Input: part model. Units: mm. Frame: model coordinates. Face numbers are marked on the shaded views. A direction names the side the tool comes from. Coordinates: 2 decimals unless noted, no trailing zeros. Order: outer loops, then holes, each group sorted by start corner. A loop starts at its lowest first (then second) coordinate and runs counter-clockwise, first axis right, second up. Notation, with made-up numbers: M 0,39.25 L 54,39.25 A11 cw 54,57.25 Z; hole C 82,60 d8. An arc over 180 degrees is marked long. Answer in a Markdown table with one row per item.
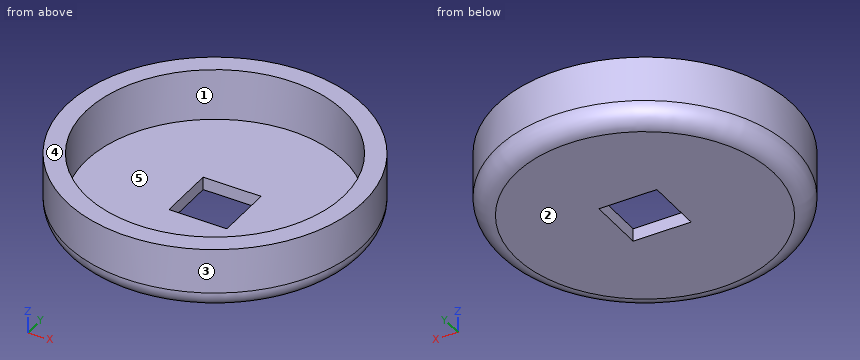
from build123d import *

# Parameters (mm, degrees)
F0_R     = 23
F0_R_2   = 20
F1_DEPTH = 10
F2_R     = 20
F2_W     = 9
F2_H     = 9
F3_DEPTH = 2
F4_R     = 3


with BuildPart() as f1:
    # F0 (on Top) → F1 (new body)
    with BuildSketch(Plane.XY):
        Circle(F0_R)
        Circle(F0_R_2, mode=Mode.SUBTRACT)
    extrude(amount=F1_DEPTH)

    # F2 (on Top) → F3 (join)
    with BuildSketch(Plane.XY):
        Circle(F2_R)
        Rectangle(F2_W, F2_H, mode=Mode.SUBTRACT)
    extrude(amount=F3_DEPTH)

    # F4
    f4_edges = [f1.edges().sort_by_distance(p)[0] for p in [
        (-23, 0, 0),
    ]]
    fillet(f4_edges, radius=F4_R)


solid = f1.part
1) Cut plane D-D, the plane z = 1.25. Output: boundary loops of the cut face in (x, y), and give its area (3 significant figures).
Resolved:
| item | result |
|---|---|
| outline | C 0,0 d44.87; hole M -4.5,-4.5 L 4.5,-4.5 L 4.5,4.5 L -4.5,4.5 Z |
| area | 1,500 mm2 |
2) Cut plane A-A, the plane y = 0. Output: boundary loops of the cut face in (x, z), and give its area (3 significant figures).
Resolved:
| item | result |
|---|---|
| outline | M -23,3 A3 ccw -20,0 L -4.5,0 L -4.5,2 L -20,2 L -20,10 L -23,10 Z; M 4.5,0 L 20,0 A3 ccw 23,3 L 23,10 L 20,10 L 20,2 L 4.5,2 Z |
| area | 118 mm2 |
3) Cut plane C-C, the plane z = 6.5. Output: boundary loops of the cut face in (x, y).
Resolved:
| item | result |
|---|---|
| outline | C 0,0 d46; hole C 0,0 d40 |
4) Mould query, pull axis Y, two halves, no side actions, for the marked faces 3, 4 and 5. Classes: +Y half, -Y half, draft (parallel to the pull), parting line (faces both ways), or undercut.
Resolved:
| item | result |
|---|---|
| face 3 | parting line |
| face 4 | draft |
| face 5 | undercut |
5) Material intervals for probe 1 along Y at (x, z) = (0, 5.5); probe 2 along Z at (x, y) = (13.5, 7.5); probe 3 along Y at (x, z) = (-10.5, 4.75), sorted ascending.
Resolved:
| item | result |
|---|---|
| probe 1 | y = -23 to -20, 20 to 23 |
| probe 2 | z = 0 to 2 |
| probe 3 | y = -20.46 to -17.02, 17.02 to 20.46 |
6) Contact query for flat-ended pins moving along their axis: pin 1 (6 mm diameter, centred on x = 15, z = 4.5, fed in from +Y); pin 2 (1 mm diameter, centred on x = -14.5, y = 18, fed in from +Z); pin 3 (6 mm diameter, centred on y = 17, z = 1, fed in from -X); pin 4 (6 mm diameter, centred on y = 6.5, z = 5.5, fed in from +X). Output: stop coordinate, or through.
Resolved:
| item | result |
|---|---|
| pin 1 | stops at y = 19.62 |
| pin 2 | stops at z = 10 |
| pin 3 | stops at x = -17.91 |
| pin 4 | stops at x = 22.73 |
7) Reachability of the marked faces 1 and 2 from +Z, -Z, +X, -X, +Y, -Y: full face, straight path, thin tool, end or side. Return the list, or none.
Resolved:
| item | result |
|---|---|
| face 1 | +Z |
| face 2 | -Z, +X, -X, +Y, -Y |
